```python
from build123d import *

# Parameters (mm, degrees)
SKETCH1_W           = 292
SKETCH1_H           = 107
BOSS_EXTRUDE1_DEPTH = 3
SKETCH2_W           = 121
SKETCH2_H           = 77
CUT_EXTRUDE2_DEPTH  = 3
SKETCH3_W           = 121
SKETCH3_H           = 77
CUT_EXTRUDE3_DEPTH  = 3
SKETCH8_W           = 3
SKETCH8_H           = 35
CUT_EXTRUDE7_DEPTH  = 3
SKETCH4_W           = 35
SKETCH4_H           = 3
BOSS_EXTRUDE2_DEPTH = 3
SKETCH7_W           = 35
SKETCH7_H           = 3
BOSS_EXTRUDE3_DEPTH = 3
SKETCH9_R           = 1.5
CUT_EXTRUDE8_DEPTH  = 10


with BuildPart() as part:
    # Sketch1 → Boss-Extrude1 (new body)
    with BuildSketch(Plane(origin=(0, 0, 0), x_dir=(1, 0, 0), z_dir=(0, 1, 0))):
        Rectangle(SKETCH1_W, SKETCH1_H)
    extrude(amount=BOSS_EXTRUDE1_DEPTH)

    # Sketch2 → Cut-Extrude2 (cut)
    with BuildSketch(Plane(origin=(0, 3, 0), x_dir=(1, 0, 0), z_dir=(0, 1, 0))):
        with Locations((-70.5, 0)):
            Rectangle(SKETCH2_W, SKETCH2_H)
    extrude(amount=-CUT_EXTRUDE2_DEPTH, mode=Mode.SUBTRACT)

    # Sketch3 → Cut-Extrude3 (cut)
    with BuildSketch(Plane(origin=(0, 3, 0), x_dir=(1, 0, 0), z_dir=(0, 1, 0))):
        with Locations((70.5, 0)):
            Rectangle(SKETCH3_W, SKETCH3_H)
    extrude(amount=-CUT_EXTRUDE3_DEPTH, mode=Mode.SUBTRACT)

    # Sketch8 → Cut-Extrude7 (cut)
    with BuildSketch(Plane(origin=(0, 3, 0), x_dir=(1, 0, 0), z_dir=(0, 1, 0))):
        with Locations((144.5, 0)):
            Rectangle(SKETCH8_W, SKETCH8_H)
        with Locations((-144.5, 0)):
            Rectangle(SKETCH8_W, SKETCH8_H)
    extrude(amount=-CUT_EXTRUDE7_DEPTH, mode=Mode.SUBTRACT)

    # Sketch4 → Boss-Extrude2 (add)
    with BuildSketch(Plane(origin=(0, 3, 0), x_dir=(1, 0, 0), z_dir=(0, 1, 0))):
        with Locations((-103.5, -55)):
            Rectangle(SKETCH4_W, SKETCH4_H)
        with Locations((-103.5, 55)):
            Rectangle(SKETCH4_W, SKETCH4_H)
        with Locations((103.5, 55)):
            Rectangle(SKETCH4_W, SKETCH4_H)
        with Locations((103.5, -55)):
            Rectangle(SKETCH4_W, SKETCH4_H)
    extrude(amount=-BOSS_EXTRUDE2_DEPTH)

    # Sketch7 → Boss-Extrude3 (add)
    with BuildSketch(Plane(origin=(0, 3, 0), x_dir=(1, 0, 0), z_dir=(0, 1, 0))):
        with Locations((0, -55)):
            Rectangle(SKETCH7_W, SKETCH7_H)
        with Locations((0, 55)):
            Rectangle(SKETCH7_W, SKETCH7_H)
    extrude(amount=-BOSS_EXTRUDE3_DEPTH)

    # Sketch9 → Cut-Extrude8 (cut)
    with BuildSketch(Plane(origin=(0, 3, 0), x_dir=(1, 0, 0), z_dir=(0, 1, 0))):
        with Locations(Location((-128.4, -42.1, 0), (0, 0, 270))):
            Circle(SKETCH9_R)
        with Locations(Location((-12.6, -42.1, 0), (0, 0, 270))):
            Circle(SKETCH9_R)
        with Locations(Location((-12.6, 42.1, 0), (0, 0, 270))):
            Circle(SKETCH9_R)
        with Locations(Location((-128.4, 42.1, 0), (0, 0, 270))):
            Circle(SKETCH9_R)
        with Locations(Location((12.6, -42.1, 0), (0, 0, 270))):
            Circle(SKETCH9_R)
        with Locations(Location((128.4, -42.1, 0), (0, 0, 270))):
            Circle(SKETCH9_R)
        with Locations(Location((128.4, 42.1, 0), (0, 0, 270))):
            Circle(SKETCH9_R)
        with Locations(Location((12.6, 42.1, 0), (0, 0, 270))):
            Circle(SKETCH9_R)
    extrude(amount=-CUT_EXTRUDE8_DEPTH, mode=Mode.SUBTRACT)


solid = part.part
```
Work out the finished part from the listing and answer in its coordinate system (mm). Coordinates: 2 decimals unless noted, no trailing zeros. Write each loop counter-clockwise with the first axis right and the second up, starting at its lowest first coordinate (ties: lowest second). Pieces come first, ordered by that corner, then holes.
Q1. A cutting plane is placed at B-B, the plane z = 27. Give the vertices of the cut face in (x, y), then the cut area to 3 significant figures.
Q2. Find the intervals of material crossed by line 1 (X direction, y = 2.45, z = -42); line 2 (X direction, y = 2.5, z = 15.5); line 3 (X direction, y = 0.2, z = -25), in increasing order.
Q3. Each of these flat-tipped pins is pushed along its axis until it touches: pin 1 Ø1.5 at (y, z) = (1, -54.5) entering from +X; pin 2 Ø0.9 at (y, z) = (1, -54.5) entering from -X; pin 3 Ø1.5 at (y, z) = (1, 4) entering from +X. Where does it stop, or does it pass through?
Q4. A cutting plane is placed at C-C, the plane y = 2.5. State how many separate pieces and enclosed holes the cut face has, then the cut area to 3 significant figures.
Q5. A cutting plane is placed at A-A, the plane x = 43. Give the vertices of the cut face in (y, z), then the cut area to 3 significant figures.
Findings below:
1. outline: (-146, 0) - (-131, 0) - (-131, 3) - (-146, 3) - close; (-10, 0) - (10, 0) - (10, 3) - (-10, 3) - close; (131, 0) - (146, 0) - (146, 3) - (131, 3) - close
1. area: 150 mm2
2. line 1: x = -146 to -129.9, -126.9 to -14.1, -11.1 to 11.1, 14.1 to 126.9, 129.9 to 146
2. line 2: x = -143 to -131, -10 to 10, 131 to 143
2. line 3: x = -146 to -131, -10 to 10, 131 to 146
3. pin 1: stops at x = 121
3. pin 2: stops at x = -121
3. pin 3: stops at x = 143
4. separate pieces: 1
4. enclosed holes: 10
4. area: 13,000 mm2
5. outline: (0, -53.5) - (3, -53.5) - (3, -38.5) - (0, -38.5) - close; (0, 38.5) - (3, 38.5) - (3, 53.5) - (0, 53.5) - close
5. area: 90.0 mm2
